Input: part model. Units: mm. Frame: model coordinates. Coordinates: 2 decimals unless noted, no trailing zeros.
1) Line query: L1, parallel to X at y = 0, z = 1; L2, parallel to X at y = -0.2, z = 1.85; L3, parallel to X at y = 1.85, z = 0.6. Output: solid intervals per line, ascending.
2) Pin query (flat end, axial travel): pin 1 Ø1.9 at (x, y) = (0, 0) entering from +Z. Return the tip coordinate at first contact, or that it passes through.
3) Section query A-A (x = 1.8). State how many separate pieces and enclosed holes the cut face has, then the cut area to 3 significant figures.
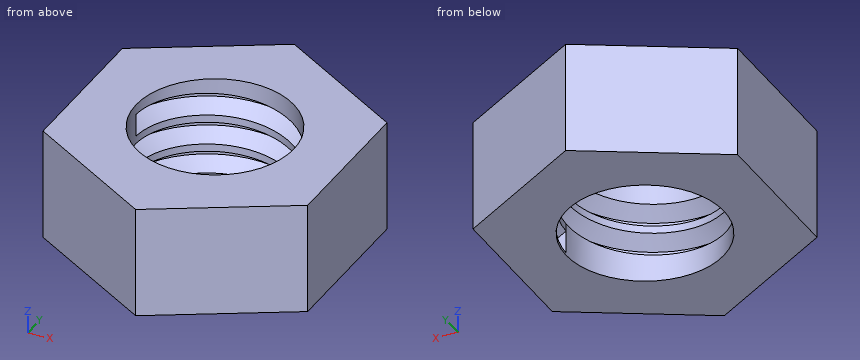
from build123d import *

# Parameters (mm, degrees)
SKETCH1_R           = 1.55
BOSS_EXTRUDE1_DEPTH = 2.2
THREAD1_PITCH       = 0.6


with BuildPart() as part:
    # Sketch1 → Boss-Extrude1 (new body)
    with BuildSketch(Plane.XY):
        Polygon((-2.598076211, -1.5), (0, -3), (2.598076211, -1.5), (2.598076211, 1.5), (0, 3), (-2.598076211, 1.5), align=None)
        Circle(SKETCH1_R, mode=Mode.SUBTRACT)
    extrude(amount=BOSS_EXTRUDE1_DEPTH)

    # Thread1: the profile of Thread Profile1 profile screwed along a right-hand helix of 2.5 turns, 6 arcs to a turn; built about Z, then put on its axis
    thread1_z = Axis((0, 0, 0), (0, 0, 1))
    thread1_corners = [(1.5497, 0, -0.000173205), (1.874759525, 0, 0.187499999), (1.874759525, 0, 0.262499999), (1.5497, 0, 0.450173203)]
    with BuildLine(mode=Mode.PRIVATE) as thread1_profile:
        Line(thread1_corners[0], thread1_corners[1])
        Line(thread1_corners[1], thread1_corners[2])
        Line(thread1_corners[2], thread1_corners[3])
        Line(thread1_corners[3], thread1_corners[0])
    thread1_cap = Face(thread1_profile.wire())
    thread1_turn_angles = [0, 30, 60, 90, 120, 150, 180, 210, 240, 270, 300, 330, 360]
    thread1_turn_weights = [1, 0.8660254037844387, 1, 0.8660254037844387, 1, 0.8660254037844387, 1, 0.8660254037844387, 1, 0.8660254037844387, 1, 0.8660254037844387, 1]
    thread1_turn_rails = [Edge.make_bspline([Vector(p[0], p[1], 0).rotate(thread1_z, thread1_turn_angles[k]) / thread1_turn_weights[k] + Vector(0, 0, p[2] + THREAD1_PITCH * thread1_turn_angles[k] / 360) for k in range(13)], [0, 0, 0, 1, 1, 2, 2, 3, 3, 4, 4, 5, 5, 6, 6, 6], 2, thread1_turn_weights) for p in thread1_corners]
    thread1_turn_sides = [Face.make_surface_from_curves(thread1_turn_rails[p[0]], thread1_turn_rails[p[1]]) for p in [(0, 1), (1, 2), (2, 3), (3, 0)]]
    thread1_last_angles = [720, 750, 780, 810, 840, 870, 900]
    thread1_last_weights = [1, 0.8660254037844387, 1, 0.8660254037844387, 1, 0.8660254037844387, 1]
    thread1_last_rails = [Edge.make_bspline([Vector(p[0], p[1], 0).rotate(thread1_z, thread1_last_angles[k]) / thread1_last_weights[k] + Vector(0, 0, p[2] + THREAD1_PITCH * thread1_last_angles[k] / 360) for k in range(7)], [0, 0, 0, 1, 1, 2, 2, 3, 3, 3], 2, thread1_last_weights) for p in thread1_corners]
    thread1_last_sides = [Face.make_surface_from_curves(thread1_last_rails[p[0]], thread1_last_rails[p[1]]) for p in [(0, 1), (1, 2), (2, 3), (3, 0)]]
    thread1 = Plane(origin=(0, 0, 2), x_dir=(-1, 0, 0), z_dir=(0, 0, -1)) * Solid(Shell([*[p.moved(Location((0, 0, THREAD1_PITCH * i))) for i in range(2) for p in thread1_turn_sides], *thread1_last_sides, thread1_cap, thread1_cap.rotate(thread1_z, 900).moved(Location((0, 0, THREAD1_PITCH * 900 / 360)))]))
    add(thread1, mode=Mode.SUBTRACT)


solid = part.part
Answer:
1. L1: x = -2.6 to -1.64, 1.72 to 2.6
1. L2: x = -2.6 to -1.54, 1.54 to 2.6
1. L3: x = -1.99 to 1.99
2. pin 1: passes through
3. separate pieces: 1
3. enclosed holes: 3
3. area: 8.28 mm2
